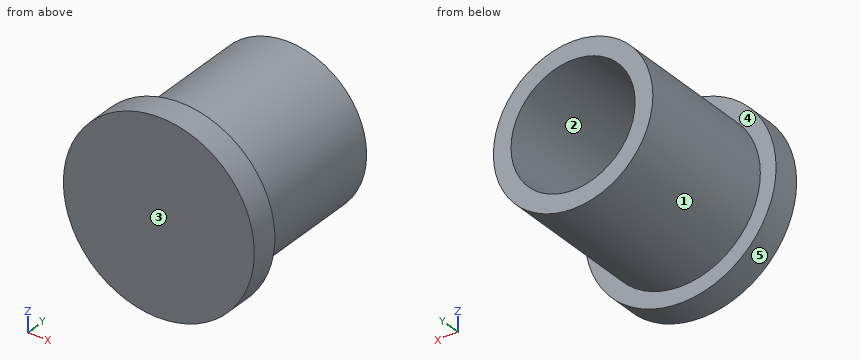
Autodesk Inventor part; units mm, degrees
ref_plane "YZ Plane" through (0, 0, 0) normal (1, 0, 0) x (0, 1, 0)
ref_plane "XZ Plane" through (0, 0, 0) normal (0, 1, 0) x (-1, 0, 0)
ref_plane "XY Plane" through (0, 0, 0) normal (0, 0, 1) x (1, 0, 0)
sketch "Esboço1" plane through (0, 0, 0) normal (0, 1, 0) x (-1, 0, 0)
  circle A0 centre (0, 0) radius 10
  dimension "d0" = 20
extrude "Extrusão1" add sketch "Esboço1" along normal blind 3
sketch "Esboço2" plane through (0, 3, 0) normal (0, 1, 0) x (1, 0, 0)
  circle A0 centre (0, 0) radius 8.35
  circle A1 centre (0, 0) radius 6.5
  dimension "d3" = 16.7
  dimension "d4" = 13
extrude "Extrusão2" add sketch "Esboço2" along normal blind 15.7
properties part number "rosca1"
Geometry: final body of the model. Coordinates: model frame, mm. Face numbers are marked on the shaded views. A direction names the side the tool comes from. Give positions to 0.01 mm unless a question says otherwise; leave off trailing zeros. Write each loop counter-clockwise with the first axis right and the second up, starting at its lowest first coordinate (ties: lowest second). Pieces come first, ordered by that corner, then holes. Notation, with made-up numbers: (-38, 82) -> (-16, 82) arc R38 ccw to (-16, 121) -> close; hole circle Ø5 at (-8.5, 49.25). An arc over 180 degrees is marked (long way). Answer as a JSON object with one key per item and string values.
1. Cut plane C-C on y = 13.25. Output: boundary loops of the cut face in (x, z).
Ans:
{"outline": "circle Ø16.7 at (0, 0); hole circle Ø13 at (0, 0)"}
2. Contact query for flat-ended pins moving along their axis: pin 1 (4 mm diameter, centred on x = 1.5, z = -0.5, fed in from +Y); pin 2 (1 mm diameter, centred on y = 8, z = 7, fed in from +X); pin 3 (5 mm diameter, centred on x = 7.5, y = 3.5, fed in from +Z). Output: stop coordinate, or through.
Ans:
{"pin 1": "stops at y = 3", "pin 2": "stops at x = 5.24", "pin 3": "stops at z = 8.63"}
3. Cut plane B-B on x = 0. Output: boundary loops of the cut face in (y, z).
Ans:
{"outline": "(0, -10) -> (3, -10) -> (3, -8.35) -> (18.7, -8.35) -> (18.7, -6.5) -> (3, -6.5) -> (3, 6.5) -> (18.7, 6.5) -> (18.7, 8.35) -> (3, 8.35) -> (3, 10) -> (0, 10) -> close"}
4. Cut plane D-D on z = 7. Output: boundary loops of the cut face in (x, y), and give its area (3 significant figures).
Ans:
{"outline": "(-7.14, 0) -> (7.14, 0) -> (7.14, 3) -> (4.55, 3) -> (4.55, 18.7) -> (-4.55, 18.7) -> (-4.55, 3) -> (-7.14, 3) -> close", "area": "186 mm^2"}
5. Mould query, pull axis X, two halves, no side actions, for the marked faces 1, 2 and 3. Classes: pulls with the +X half, pulls with the -X half, needs draft (parallel to the pull), parting line crosses it, or undercut.
Ans:
{"face 1": "parting line crosses it", "face 2": "undercut", "face 3": "needs draft"}
6. Ray query, probe 1 along X at (y, z) = (9.25, 0); probe 2 along Y at (x, z) = (1.75, 1). Return the intervals inside material, ascending. Write a range as from..to.
Ans:
{"probe 1": "x = -8.35..-6.5, 6.5..8.35", "probe 2": "y = 0..3"}
7. Cut plane A-A on z = 0. Output: boundary loops of the cut face in (x, y), and give its area (3 significant figures).
Ans:
{"outline": "(-10, 0) -> (10, 0) -> (10, 3) -> (8.35, 3) -> (8.35, 18.7) -> (6.5, 18.7) -> (6.5, 3) -> (-6.5, 3) -> (-6.5, 18.7) -> (-8.35, 18.7) -> (-8.35, 3) -> (-10, 3) -> close", "area": "118 mm^2"}
8. Access query for the marked faces 4 and 5. Directions: +Z, -Z, +X, -X, +Y, -Y. A direction counts if a zero-diameter tool reaches every point of the face in a straight line with its end or side. Return the directions, or none.
Ans:
{"face 4": "+Y", "face 5": "+Y, -Y"}
